CAD build for the part. Positions are in the model's coordinates, mm. A direction names the side the tool comes from. Give positions to 0.01 mm unless a question says otherwise; leave off trailing zeros. Loops run counter-clockwise (first coordinate to the right, second up) from the corner with the lowest first, then second, coordinate; pieces in that order, holes last. Notation, with made-up numbers: M -11,59 L 19,59 A12 ccw 19,82 Z; hole C 18.25,-31.5 d6. An arc over 180 degrees is marked long. Answer as CSV lines item,"result".
from build123d import *

# Parameters (mm, degrees)
SCHIZZO1_W                    = 26
SCHIZZO1_H                    = 17.22
ESTRUSIONE_ESTRUSIONE1_DEPTH  = 5.08
TAGLIO_ESTRUSIONE1_DEPTH      = 17.399344499
FORO_FILETTATO_M3X0_5_1_D     = 2.5
FORO_FILETTATO_M3X0_5_1_DEPTH = 8
FORO_FILETTATO_M3X0_5_1_TIP   = 0.751075774


with BuildPart() as part:
    # Schizzo1 → Estrusione-Estrusione1 (new body)
    with BuildSketch(Plane.XY):
        Rectangle(SCHIZZO1_W, SCHIZZO1_H)
    extrude(amount=-ESTRUSIONE_ESTRUSIONE1_DEPTH)

    # Schizzo2 → Taglio-Estrusione1 (cut, through all)
    with BuildSketch(Plane.XY):
        Polygon((-9.5, 8.61), (9.5, 8.61), (8.07, 6.65), (-8.07, 6.65), align=None)
    extrude(amount=-TAGLIO_ESTRUSIONE1_DEPTH, mode=Mode.SUBTRACT)

    # Foro filettato M3x0.5-1
    with Locations(Plane(origin=(0, -8.61, 0), x_dir=(-1, 0, 0), z_dir=(0, -1, 0))):
        with Locations((10, 2.54), (-10, 2.54)):
            Hole(FORO_FILETTATO_M3X0_5_1_D / 2, depth=FORO_FILETTATO_M3X0_5_1_DEPTH)
            with Locations((0, 0, -(FORO_FILETTATO_M3X0_5_1_DEPTH + FORO_FILETTATO_M3X0_5_1_TIP / 2))):  # 118° drill point
                Cone(0, FORO_FILETTATO_M3X0_5_1_D / 2, FORO_FILETTATO_M3X0_5_1_TIP, mode=Mode.SUBTRACT)

    # Schizzo5 → Foro filettato M3x0.5-2 (revolve, cut)
    with BuildSketch(Plane(origin=(-13, 4.39, -2.54), x_dir=(0, 0, 1), z_dir=(0, 1, 0))):
        Polygon((0, 0), (0, 6.751075774), (1.25, 6), (1.25, 0), align=None)
    foro_filettato_m3x0_5_2 = revolve(axis=Axis((-19.35, 4.39, -2.54), (1, 0, 0)), mode=Mode.SUBTRACT)

    # Specchia1: Foro filettato M3x0.5-2 across plane
    add(foro_filettato_m3x0_5_2.mirror(Plane(origin=(0, 0, 0), x_dir=(0, 0, 1), z_dir=(1, 0, 0))), mode=Mode.SUBTRACT)


solid = part.part
1) Band-saw the part on B-B on y = -2. Give the cut face in (x, z).
Answer below:
outline,"M -13,-5.08 L 13,-5.08 L 13,0 L -13,0 Z; hole C -10,-2.54 d2.5; hole C 10,-2.54 d2.5"
2) Mould opens along Z. For faces 1 (the face through (6.38, 4.21, -2.42)), 2 (the face through (0, 0, -5.08)), 3 (the face through (8.795, 7.644, -2.504)) say: +Z half, -Z half, draft (parallel to the pull), parting line (faces both ways), or undercut.
Answer below:
face 1,"undercut"
face 2,"-Z half"
face 3,"draft"
3) Flat gauge pin, fed straight in: pin 1 (1.5 mm diameter, centred on x = 10, z = -2.54, fed in from -Y). Where does the tip first touch, or does it go through?
Answer below:
pin 1,"stops at y = -0.31"
4) Drill centre lines: line 1 (Z direction, x = 8.65, y = 4.39); line 2 (X direction, y = -5, z = -3.35); line 3 (Y direction, x = -3.5, z = -2.4). Where is each one in solid material? Low to high. Write a range as from..to.
Answer below:
line 1,"z = -5.08..-3.79, -1.29..0"
line 2,"x = -13..-10.95, -9.05..9.05, 10.95..13"
line 3,"y = -8.61..6.65"
5) Band-saw the part on C-C on x = -3. Give the cut face in (y, z), and give its area (3 significant figures).
Answer below:
outline,"M -8.61,-5.08 L 6.65,-5.08 L 6.65,0 L -8.61,0 Z"
area,"77.5 mm^2"
6) Band-saw the part on A-A on z = -0.35. Give the cut face in (x, y), and give its area (3 significant figures).
Answer below:
outline,"M -13,-8.61 L 13,-8.61 L 13,8.61 L 9.5,8.61 L 8.07,6.65 L -8.07,6.65 L -9.5,8.61 L -13,8.61 Z"
area,"413 mm^2"
7) Which spindle directions (+Z, -Z, +X, -X, +Y, -Y) get a long thin tool onto all of the face, cutting with end or side? Do faces 4 (the face through (10.04, 5.15, -3.53)), 5 (the face through (-10.04, 5.15, -3.53)), 6 (the face through (0, 6.65, -3)), 7 (the face through (9.01, -4.55, -1.78)), 8 (the face through (13, 0, -3)). Say none if no direction does.
Answer below:
face 4,"+X"
face 5,"-X"
face 6,"+Z, -Z, +Y"
face 7,"-Y"
face 8,"+Z, -Z, +X, +Y, -Y"
